Geometry check sheet. Reference: drawing and pictorial views, mm from the part's lowest x, y, z. Round coordinates to 2 decimals unless told otherwise and drop trailing zeros. Write each loop counter-clockwise with the first axis right and the second up, starting at its lowest first coordinate (ties: lowest second). Pieces come first, ordered by that corner, then holes. Notation, with made-up numbers: M 24,-7.5 L 67,-7.5 A17 cw 67,24.5 Z; hole C 35,48.5 d5. An arc over 180 degrees is marked long. One line per item, written item: value. Start each with the question number.
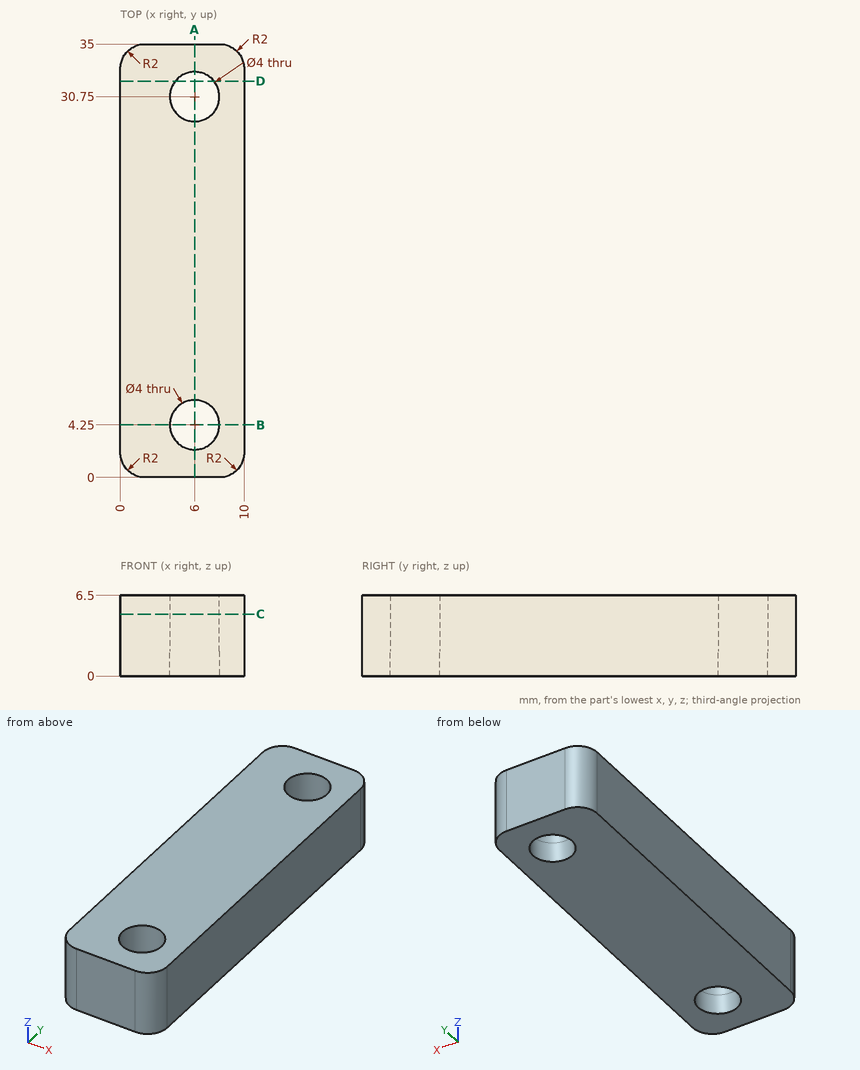
1) Cross-section at B-B (y = 4.25). Record the boundary of the cut face in (x, z).
2) Cross-section at C-C (z = 5). Record the boundary of the cut face in (x, y).
3) Thickness scan on line 1 (Y direction, x = 6, z = 0.4); line 2 (Y direction, x = 4.75, z = 0.75); line 3 (X direction, y = 31, z = 6). Record the ranges inside material, lowest first.
4) Cross-section at D-D (y = 32). Record the boundary of the cut face in (x, z), then the cut area to 3 significant figures.
5) Cross-section at A-A (x = 6). Record the boundary of the cut face in (y, z), then the cut area to 4 significant figures.
Results below:
1. outline: M 0,0 L 4,0 L 4,6.5 L 0,6.5 Z; M 8,0 L 10,0 L 10,6.5 L 8,6.5 Z
2. outline: M 0,2 A2 ccw 2,0 L 8,0 A2 ccw 10,2 L 10,33 A2 ccw 8,35 L 2,35 A2 ccw 0,33 Z; hole C 6,4.25 d4; hole C 6,30.75 d4
3. line 1: y = 0 to 2.25, 6.25 to 28.75, 32.75 to 35
3. line 2: y = 0 to 2.69, 5.81 to 29.19, 32.31 to 35
3. line 3: x = 0 to 4.02, 7.98 to 10
4. outline: M 0,0 L 4.44,0 L 4.44,6.5 L 0,6.5 Z; M 7.56,0 L 10,0 L 10,6.5 L 7.56,6.5 Z
4. area: 44.7 mm²
5. outline: M 0,0 L 2.25,0 L 2.25,6.5 L 0,6.5 Z; M 6.25,0 L 28.75,0 L 28.75,6.5 L 6.25,6.5 Z; M 32.75,0 L 35,0 L 35,6.5 L 32.75,6.5 Z
5. area: 175.5 mm²
